Here's the drawing with two shaded views (mm, measured from the low corner). I have some questions. A direction names the side the tool comes from. Round coordinates to 2 decimals unless told otherwise and drop trailing zeros. Loops run counter-clockwise (first coordinate to the right, second up) from the corner with the lowest first, then second, coordinate; pieces in that order, holes last.
(1) Thinking about a two-plate mould opening in X: for the marked faces 1, 2 and 3, which applies, released by +X, released by -X, zero draft, split by the parting line, or undercut?
(2) Which directions (+Z, -Z, +X, -X, +Y, -Y) give clear straight access to the entire face, cutting with the end or side of a thin tool? Please do the marked faces 4 and 5.
(3) I want a section at B-B on z = 19.75. Write out the boundary of the cut face in (x, y).
(4) Will these pins go through, and if not, where does the flat tip stop? pin 1 Ø12.5 at (y, z) = (114.5, 12.5) entering from +X; pin 2 Ø1 at (x, z) = (13, 15) entering from +Y; pin 3 Ø5.5 at (y, z) = (161.925, 12.7) entering from +X.
(5) I want a section at A-A on y = 114.3. Write out the boundary of the cut face in (x, z), plus the area to 3 significant figures.
(6) If I drill on line 1 along Y through (x, z) = (52.75, 12.7); line 2 along X through (y, z) = (1.75, 12.7); line 3 along Z through (x, y) = (52, 209.55), over which ranges is the centre line in solid material (lowest first)?
(7) I want a section at C-C on x = 21. Write out the boundary of the cut face in (y, z), plus the area to 3 significant figures.
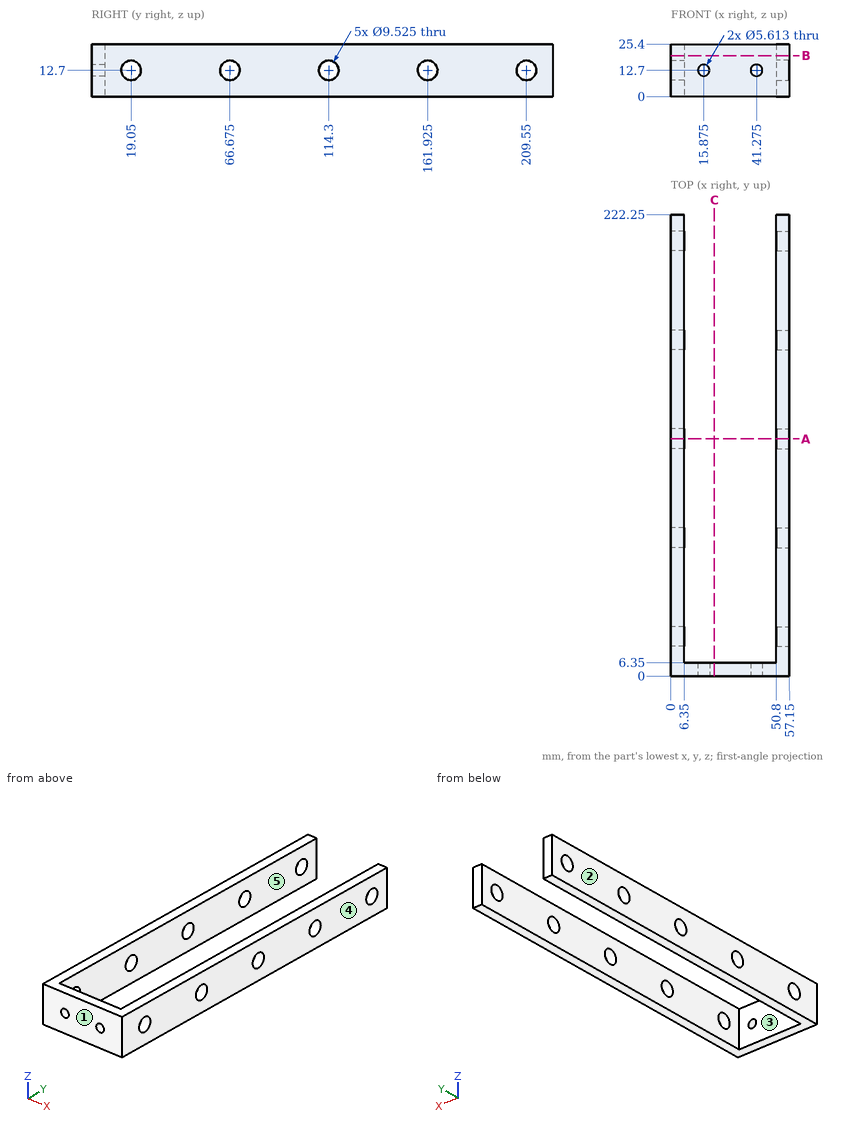
Filled sheet:
1. face 1: zero draft
1. face 2: released by -X
1. face 3: undercut
2. face 4: +Z, -Z, +X, +Y, -Y
2. face 5: +Z, -Z, +Y
3. outline: (0, 0) - (57.15, 0) - (57.15, 222.25) - (50.8, 222.25) - (50.8, 6.35) - (6.35, 6.35) - (6.35, 222.25) - (0, 222.25) - close
4. pin 1: stops at x = 57.15
4. pin 2: stops at y = 6.35
4. pin 3: passes through
5. outline: (0, 0) - (6.35, 0) - (6.35, 7.94) - (0, 7.94) - close; (0, 17.46) - (6.35, 17.46) - (6.35, 25.4) - (0, 25.4) - close; (50.8, 0) - (57.15, 0) - (57.15, 7.94) - (50.8, 7.94) - close; (50.8, 17.46) - (57.15, 17.46) - (57.15, 25.4) - (50.8, 25.4) - close
5. area: 202 mm2
6. line 1: y = 0 to 14.29, 23.81 to 61.91, 71.44 to 109.54, 119.06 to 157.16, 166.69 to 204.79, 214.31 to 222.25
6. line 2: x = 0 to 13.07, 18.68 to 38.47, 44.08 to 57.15
6. line 3: z = 0 to 7.94, 17.46 to 25.4
7. outline: (0, 0) - (6.35, 0) - (6.35, 25.4) - (0, 25.4) - close
7. area: 161 mm2
